Design review of the part built by this model. Coordinates are the model's own, in mm. Give positions to 0.01 mm unless a question says otherwise; leave off trailing zeros. Order: outer loops, then holes, each group sorted by start corner. A loop starts at its lowest first (then second) coordinate and runs counter-clockwise, first axis right, second up. Notation, with made-up numbers: M 79,26.25 L 83,26.25 A21 ccw 83,60.25 Z; hole C 29,7.25 d1. An arc over 180 degrees is marked long. Answer as a JSON object with one key per item and string values.
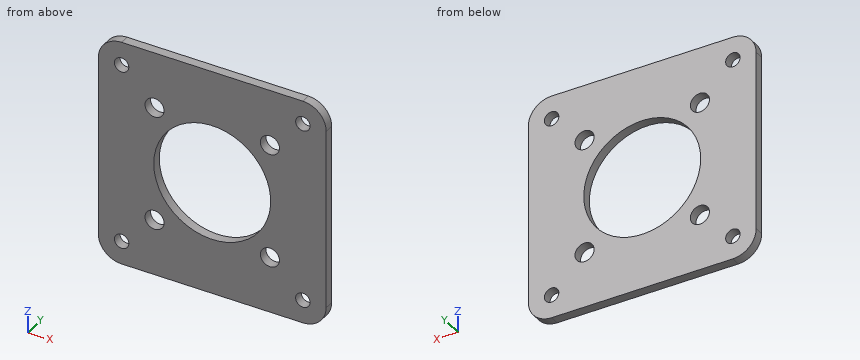
Autodesk Inventor part; units mm, degrees
ref_plane "YZ Plane" through (0, 0, 0) normal (1, 0, 0) x (0, 1, 0)
ref_plane "XZ Plane" through (0, 0, 0) normal (0, 1, 0) x (-1, 0, 0)
ref_plane "XY Plane" through (0, 0, 0) normal (0, 0, 1) x (1, 0, 0)
sketch "スケッチ1" plane through (0, 0, 0) normal (0, 1, 0) x (-1, 0, 0)
  circle A0 centre (0, 0) radius 12.55
  line L0 (0, 0) -> (0, -12.55) construction
  circle A1 centre (12.3744, -12.3744) radius 2.05
  line L1 (0, 0) -> (8.8742, -8.8742) construction
  circle A2 centre (19.4454, -19.4454) radius 1.55
  circle A3 centre (0, 0) radius 27.5 construction
  circle A4 centre (19.4454, 19.4454) radius 1.55
  circle A5 centre (-19.4454, 19.4454) radius 1.55
  circle A6 centre (-19.4454, -19.4454) radius 1.55
  line L2 (-24.4454, 24.4454) -> (24.4454, 24.4454)
  line L3 (24.4454, 24.4454) -> (24.4454, -24.4454)
  line L4 (24.4454, -24.4454) -> (-24.4454, -24.4454)
  line L5 (-24.4454, -24.4454) -> (-24.4454, 24.4454)
  line L6 (-24.4454, 24.4454) -> (24.4454, -24.4454) construction
  line L7 (24.4454, 24.4454) -> (-24.4454, -24.4454) construction
  circle A7 centre (12.3744, 12.3744) radius 2.05
  circle A8 centre (-12.3744, 12.3744) radius 2.05
  circle A9 centre (-12.3744, -12.3744) radius 2.05
  dimension "d9" = 55
  dimension "d0" = 25.1
  dimension "d1" = 4.1
  dimension "d7" = 45
  dimension "d8" = 3.1
  dimension "d12" = 360
  dimension "d14" = 5
  dimension "d20" = 360
  dimension "d22" = 35
extrude "押し出し1" add sketch "スケッチ1" along normal blind 2
fillet "フィレット1" radius 5 4 edges at (24.4454, 1, 24.4454) (24.4454, 1, -24.4454) (-24.4454, 1, -24.4454) (-24.4454, 1, 24.4454)
sketch "スケッチ2" plane through (0, 2, 0) normal (0, 1, 0) x (1, 0, 0)
  arc A0 (-24.4454, -19.4454) -> (-19.4454, -24.4454) centre (-19.4454, -19.4454) ccw
  line L0 (-19.4454, -24.4454) -> (19.4454, -24.4454)
  arc A1 (19.4454, -24.4454) -> (24.4454, -19.4454) centre (19.4454, -19.4454) ccw
  line L1 (24.4454, -19.4454) -> (24.4454, 19.4454)
  arc A2 (24.4454, 19.4454) -> (19.4454, 24.4454) centre (19.4454, 19.4454) ccw
  line L2 (19.4454, 24.4454) -> (-19.4454, 24.4454)
  arc A3 (-19.4454, 24.4454) -> (-24.4454, 19.4454) centre (-19.4454, 19.4454) ccw
  line L3 (-24.4454, 19.4454) -> (-24.4454, -19.4454)
  circle A4 centre (-19.4454, 19.4454) radius 1.55
  circle A5 centre (-19.4454, -19.4454) radius 1.55
  circle A6 centre (19.4454, -19.4454) radius 1.55
  circle A7 centre (19.4454, 19.4454) radius 1.55
  circle A8 centre (12.3744, 12.3744) radius 2.05
  circle A9 centre (12.3744, -12.3744) radius 2.05
  circle A10 centre (-12.3744, -12.3744) radius 2.05
  circle A11 centre (-12.3744, 12.3744) radius 2.05
  circle A12 centre (0, 0) radius 12.55
properties part number "omu_al_jo_2" material "アルミニウム 6061-AHC"
(1) To check wall thickness, follow L1, parallel to Z at x = 20, y = 0.15; L2, parallel to Z at x = 0, y = 0.9; L3, parallel to Z at x = 14, y = 1.35. State the ranges of each line that lie inside material, in increasing order. Write a range as from..to.
Checked values:
{"L1": "z = -24.41..-20.89, -18..18, 20.89..24.41", "L2": "z = -24.45..-12.55, 12.55..24.45", "L3": "z = -24.45..-13.62, -11.13..11.13, 13.62..24.45"}
(2) We need section A-A (x = 0). Write out the cut boundary in (y, z).
Checked values:
{"outline": "M 0,-24.45 L 2,-24.45 L 2,-12.55 L 0,-12.55 Z; M 0,12.55 L 2,12.55 L 2,24.45 L 0,24.45 Z"}
(3) We need section C-C (y = 1.5). Count the separate pieces of the cut face and the enclosed holes in it, plus the area to 3 significant figures.
Checked values:
{"separate pieces": "1", "enclosed holes": "9", "area": "1,790 mm^2"}
(4) We need section B-B (z = 0). Write out the cut boundary in (x, y).
Checked values:
{"outline": "M -24.45,0 L -12.55,0 L -12.55,2 L -24.45,2 Z; M 12.55,0 L 24.45,0 L 24.45,2 L 12.55,2 Z"}
(5) Insertion check: pin 1 (3.5 mm diameter, centred on x = 12.37, z = -12.37, fed in from +Y). The pin has a flat end and moves straight along its axis. Give the tip position at first contact, or say it passes through.
Checked values:
{"pin 1": "passes through"}
